Build history of the part. All positions in model axes, mm. Face numbers are marked on the shaded views. Round coordinates to 2 decimals unless told otherwise and drop trailing zeros. Loops run counter-clockwise (first coordinate to the right, second up) from the corner with the lowest first, then second, coordinate; pieces in that order, holes last. Notation, with made-up numbers: (67, 29) -> (116, 29) arc R23 ccw to (116, 40) -> close; hole circle Ø3 at (34, 20). An arc over 180 degrees is marked (long way). Put each result on its own line as item: value. Start each with the question number.
```python
from build123d import *

# Parameters (mm, degrees)
SKETCH_1_W          = 52
SKETCH_1_H          = 28
EXTRUDE_1_DEPTH     = 6
SKETCH_2_W          = 50
SKETCH_2_H          = 26
CUT_EXTRUDE_1_DEPTH = 5
SKETCH_3_W          = 1
SKETCH_3_H          = 26
CUT_EXTRUDE_2_DEPTH = 4
CUT_EXTRUDE_3_REACH = 56.185
SKETCH_6_R          = 1.5
CUT_EXTRUDE_4_DEPTH = 4
EXTRUDE_START       = 3
SKETCH_7_R          = 2.5
SKETCH_7_R_2        = 1.5
SKETCH_7_R_3        = 1
EXTRUDE_3_DEPTH     = 3
CHAMFER_2_SIZE      = 2
CHAMFER_3_SIZE      = 3.5
CHAMFER_3_SIZE2     = 2
FILLET_1_R          = 0.5
FILLET_2_R          = 0.5
EXTRUDE_4_REACH     = 32.799
EXTRUDE_START_2     = -1
SKETCH_9_W          = 0.8
SKETCH_9_H          = 2
CUT_EXTRUDE_5_DEPTH = 1
CHAMFER_4_SIZE      = 1
CHAMFER_4_SIZE_2    = 0.1


# Some blends are built 0.0001 mm under size
with BuildPart() as part:
    # Эскиз1 → Бобышка-Вытянуть1 (new body)
    with BuildSketch(Plane(origin=(0, 0, 0), x_dir=(1, 0, 0), z_dir=(0, 1, 0))):
        Rectangle(SKETCH_1_W, SKETCH_1_H)
    extrude(amount=EXTRUDE_1_DEPTH)

    # Эскиз2 → Вырез-Вытянуть1 (cut)
    with BuildSketch(Plane(origin=(0, 6, 0), x_dir=(1, 0, 0), z_dir=(0, 1, 0))):
        Rectangle(SKETCH_2_W, SKETCH_2_H)
    extrude(amount=-CUT_EXTRUDE_1_DEPTH, mode=Mode.SUBTRACT)

    # Эскиз3 → Вырез-Вытянуть2 (cut)
    with BuildSketch(Plane(origin=(0, 6, 0), x_dir=(1, 0, 0), z_dir=(0, 1, 0))):
        with Locations((25.5, 0)):
            Rectangle(SKETCH_3_W, SKETCH_3_H)
    extrude(amount=-CUT_EXTRUDE_2_DEPTH, mode=Mode.SUBTRACT)

    # Эскиз4 → Вырез-Вытянуть3 (cut, up to next)
    with BuildSketch(Plane.ZY.offset(26), mode=Mode.PRIVATE) as cut_extrude_3_sk1:
        with BuildLine():
            Line((-2.5, 8), (2.5, 8))
            ThreePointArc((2.5, 8), (4, 6.5), (2.5, 5))
            Line((2.5, 5), (-2.5, 5))
            ThreePointArc((-2.5, 5), (-4, 6.5), (-2.5, 8))
        make_face()
    cut_extrude_3_tool1 = extrude(cut_extrude_3_sk1.sketch, amount=-CUT_EXTRUDE_3_REACH, mode=Mode.PRIVATE) & part.part
    add(cut_extrude_3_tool1.solids().sort_by_distance((-26, 6.5, 0))[0], mode=Mode.SUBTRACT)

    # Эскиз6 → Вырез-Вытянуть4 (cut)
    with BuildSketch(Plane(origin=(0, 1, 0), x_dir=(1, 0, 0), z_dir=(0, 1, 0))):
        with Locations(Location((-18.5, 9.5, 0), (0, 0, 270))):
            Circle(SKETCH_6_R)
    extrude(amount=-CUT_EXTRUDE_4_DEPTH, mode=Mode.SUBTRACT)

    # Эскиз7 → Бобышка-Вытянуть3 (add)
    # profile 1 of 2: a face of its own
    with BuildSketch(Plane(origin=(0, 1, 0), x_dir=(1, 0, 0), z_dir=(0, 1, 0)).offset(EXTRUDE_START)):
        with Locations(Location((-18.5, 9.5, 0), (0, 0, 270))):
            Circle(SKETCH_7_R)
        with Locations(Location((-18.5, 9.5, 0), (0, 0, 270))):
            Circle(SKETCH_7_R_2, mode=Mode.SUBTRACT)
    # profile 2 of 2: a face of its own
    with BuildSketch(Plane(origin=(0, 1, 0), x_dir=(1, 0, 0), z_dir=(0, 1, 0)).offset(EXTRUDE_START)):
        with Locations(Location((-23, -11, 0), (0, 0, 270))):
            Circle(SKETCH_7_R_3)
    extrude(amount=-EXTRUDE_3_DEPTH)

    # Фаска2
    # the kernel refuses this chamfer: 2 mm, written as the material it adds along each edge
    with BuildSketch(Plane(origin=(-18.5, 1, -9.5), x_dir=(0, 0, 1), z_dir=(-1, 0, 0))) as chamfer_2_piece_1:
        Polygon((2.5 + CHAMFER_2_SIZE, 0), (2.5, CHAMFER_2_SIZE), (2.5, 0), align=None)
    revolve(axis=Axis((-18.5, 1, -9.5), (0, 1, 0)))

    # Фаска3
    chamfer_3_edges = [part.edges().sort_by_distance(p)[0] for p in [
        (-18.5, 0, -11),
    ]]
    chamfer_3_side = [part.faces().sort_by_distance(p)[0] for p in [
        (-18.5, 2, -11),
    ]]
    chamfer(chamfer_3_edges, length=CHAMFER_3_SIZE, length2=CHAMFER_3_SIZE2, reference=chamfer_3_side[0])

    # Скругление1
    fillet_1_edges = [part.edges().sort_by_distance(p)[0] for p in [
        (-25, 1, 0),
        (4.664213562, 1, -13),
        (-23.164213562, 1, -13),
        (25, 1, 0),
        (0, 1, 13),
        (-22.742640687, 1, -8),
        (0, 0, -14),
        (-26, 0, 0),
        (0, 0, 14),
        (26, 0, 0),
        (-18.5, 0, -13),
        (-18.5, 4, -12),
        (-18.5, 3, -12),
        (25, 1.5, -13),
        (25, 1.5, 13),
        (26, 3, -14),
        (-26, 3, -14),
        (-26, 3, 14),
        (-18.5, 3.5, -11),
    ]]
    fillet(fillet_1_edges, radius=FILLET_1_R)

    # Скругление2
    fillet_2_edges = [part.edges().sort_by_distance(p)[0] for p in [
        (-23, 1, 10),
    ]]
    fillet(fillet_2_edges, radius=FILLET_2_R - 0.0001)  # a hair under: the kernel refuses the full size

    # Эскиз9 → Бобышка-Вытянуть4 (add, up to next)
    with BuildSketch(Plane(origin=(0, 4, 0), x_dir=(1, 0, 0), z_dir=(0, 1, 0)).offset(EXTRUDE_START_2), mode=Mode.PRIVATE) as extrude_4_sk1:
        with Locations((-23, -12)):
            Rectangle(SKETCH_9_W, SKETCH_9_H)
    extrude_4_tool1 = extrude(extrude_4_sk1.sketch, amount=-EXTRUDE_4_REACH, mode=Mode.PRIVATE) - part.part
    # Эскиз9 → Бобышка-Вытянуть4 (add, up to next)
    with BuildSketch(Plane(origin=(0, 4, 0), x_dir=(1, 0, 0), z_dir=(0, 1, 0)).offset(EXTRUDE_START_2), mode=Mode.PRIVATE) as extrude_4_sk2:
        Polygon((-25, -11), (-25, -11.4), (-23, -11.4), (-23, -11), (-23, -10.6), (-25, -10.6), align=None)
    extrude_4_tool2 = extrude(extrude_4_sk2.sketch, amount=-EXTRUDE_4_REACH, mode=Mode.PRIVATE) - part.part
    add(extrude_4_tool1.solids().sort_by_distance((-23, 3, 12))[0])
    add(extrude_4_tool2.solids().sort_by_distance((-24, 3, 11))[0])

    # Эскиз10 → Вырез-Вытянуть5 (cut)
    with BuildSketch(Plane(origin=(0, 6, 0), x_dir=(1, 0, 0), z_dir=(0, 1, 0))):
        Polygon((26, 13), (26, 13.5), (-25.5, 13.5), (-25.5, -13.5), (26, -13.5), (26, -13), (-25, -13), (-25, 13), align=None)
    extrude(amount=-CUT_EXTRUDE_5_DEPTH, mode=Mode.SUBTRACT)

    # Фаска4
    # the kernel refuses this chamfer: 1, 0.1 mm, written as the material it takes off along each edge
    with BuildSketch(Plane(origin=(-25.5, 6, -16.099522763), x_dir=(0, -1, 0), z_dir=(0, 0, 1))) as chamfer_4_piece_1_section:
        Polygon((CHAMFER_4_SIZE, 0), (0, -CHAMFER_4_SIZE_2), (0, 0), align=None)
    chamfer_4_piece_1 = extrude(amount=14.784831964, mode=Mode.PRIVATE)
    chamfer_4_piece_1 = split(chamfer_4_piece_1, bisect_by=Plane(origin=(-25.5, 6.247477501, -13.62474775), z_dir=(0, 0.09950371902099857, 0.9950371902099893)), keep=Keep.TOP, mode=Mode.PRIVATE)
    add(chamfer_4_piece_1, mode=Mode.SUBTRACT)
    with BuildSketch(Plane(origin=(28.599522763, 6, -13.5), x_dir=(0, -1, 0), z_dir=(-1, 0, 0))) as chamfer_4_piece_2_section:
        Polygon((CHAMFER_4_SIZE, 0), (0, -CHAMFER_4_SIZE_2), (0, 0), align=None)
    chamfer_4_piece_2 = extrude(amount=56.699045526, mode=Mode.PRIVATE)
    chamfer_4_piece_2 = split(chamfer_4_piece_2, bisect_by=Plane(origin=(-25.063371062, 0.633710618, -13.5), z_dir=(0.995037190209989, 0.09950371902100032, 0)), keep=Keep.TOP, mode=Mode.PRIVATE)
    add(chamfer_4_piece_2, mode=Mode.SUBTRACT)
    with BuildSketch(Plane(origin=(-28.099522763, 6, 13.5), x_dir=(0, -1, 0), z_dir=(1, 0, 0))) as chamfer_4_piece_3_section:
        Polygon((CHAMFER_4_SIZE, 0), (0, -CHAMFER_4_SIZE_2), (0, 0), align=None)
    chamfer_4_piece_3 = extrude(amount=56.699045526, mode=Mode.PRIVATE)
    chamfer_4_piece_3 = split(chamfer_4_piece_3, bisect_by=Plane(origin=(-25.62474775, 6.247477501, 13.5), z_dir=(0.995037190209989, 0.09950371902100032, 0)), keep=Keep.TOP, mode=Mode.PRIVATE)
    add(chamfer_4_piece_3, mode=Mode.SUBTRACT)
    with BuildSketch(Plane(origin=(-25.5, 6, 1.314690799), x_dir=(0, -1, 0), z_dir=(0, 0, 1))) as chamfer_4_piece_4_section:
        Polygon((CHAMFER_4_SIZE, 0), (0, -CHAMFER_4_SIZE_2), (0, 0), align=None)
    chamfer_4_piece_4 = extrude(amount=14.784831964, mode=Mode.PRIVATE)
    chamfer_4_piece_4 = split(chamfer_4_piece_4, bisect_by=Plane(origin=(-25.5, 4.783632752, 13.478363275), z_dir=(0, 0.09950371902099857, -0.9950371902099893)), keep=Keep.TOP, mode=Mode.PRIVATE)
    add(chamfer_4_piece_4, mode=Mode.SUBTRACT)


solid = part.part
```
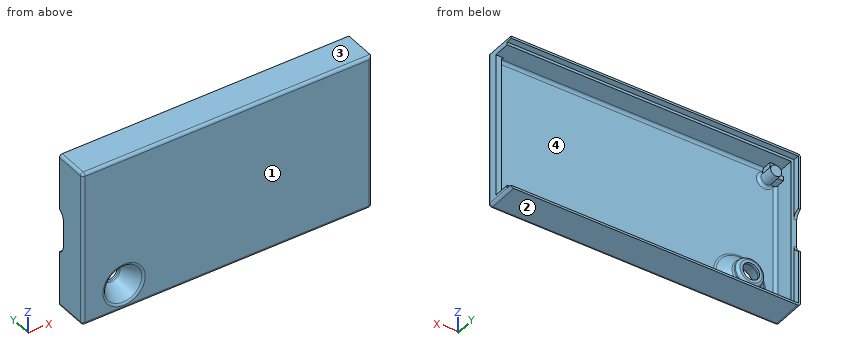
Item 1: Wall check: line 1 (Z direction, x = -10, y = 2.5); line 2 (X direction, y = 3.9, z = -9.5); line 3 (X direction, y = 1.75, z = 9.25). Give the ranges that are in metal, low to high. Write a range as from..to.
Item 2: Cut at B-B on x = -11.5. Write the cut outline in (y, z), then the cut area to 3 significant figures.
Item 3: Cut at D-D on z = 9. Write the cut outline in (x, y).
Item 4: Drop flat-ended pins along their axis: pin 1 (4.5 mm diameter, centred on x = -18, z = -8.5, fed in from +Y); pin 2 (4 mm diameter, centred on x = 12.5, z = 3, fed in from +Y); pin 3 (0.9 mm diameter, centred on x = -23, z = 12.5, fed in from +Y). Give the stop position or say it passes through.
Item 5: Pull direction Z, two halves, no side cores. Call the marked faces 1, 2, 3 and 4: +Z half, -Z half, draft (parallel to the pull), parting line (faces both ways), or undercut.
Item 6: Cut at C-C on z = -0.5. Write the cut outline in (x, y).
Item 7: Cut at A-A on y = 5.5. Write the cut outline in (x, z).
Ans:
1. line 1: z = -14..-13, 13..14
1. line 2: x = -26..-25, -20.8..-20, -17..-16.2
1. line 3: x = -26..-25, 25..26
2. outline: (0, -13.5) arc R0.5 ccw to (0.5, -14) -> (6, -14) -> (6, -13.6) -> (5, -13.5) -> (5, -13) -> (1.5, -13) arc R0.5 cw to (1, -12.5) -> (1, 12.5) arc R0.5 cw to (1.5, 13) -> (5, 13) -> (5, 13.5) -> (6, 13.6) -> (6, 14) -> (0.5, 14) arc R0.5 ccw to (0, 13.5) -> close
2. area: 36.9 mm2
3. outline: (-26, 0.5) arc R0.5 ccw to (-25.5, 0) -> (25.5, 0) arc R0.5 ccw to (26, 0.5) -> (26, 2) -> (25, 2) -> (25, 1.5) arc R0.5 cw to (24.5, 1) -> (-24.5, 1) arc R0.5 cw to (-25, 1.5) -> (-25, 5) -> (-25.5, 5) -> (-25.6, 6) -> (-26, 6) -> close
4. pin 1: stops at y = 4
4. pin 2: stops at y = 1
4. pin 3: stops at y = 3
5. face 1: draft
5. face 2: -Z half
5. face 3: +Z half
5. face 4: undercut
6. outline: (-26, 0.5) arc R0.5 ccw to (-25.5, 0) -> (25.5, 0) arc R0.5 ccw to (26, 0.5) -> (26, 2) -> (25, 2) -> (25, 1.5) arc R0.5 cw to (24.5, 1) -> (-24.5, 1) arc R0.5 cw to (-25, 1.5) -> (-25, 5) -> (-26, 5) -> close
7. outline: (-26, -13.5) arc R0.5 ccw to (-25.5, -14) -> (25.5, -14) arc R0.5 ccw to (26, -13.55) -> (-25.55, -13.55) -> (-25.55, -3.62) -> (-26, -3.62) -> close; (-26, 3.62) -> (-25.55, 3.62) -> (-25.55, 13.55) -> (26, 13.55) -> (26, 14) -> (-25.5, 14) arc R0.5 ccw to (-26, 13.5) -> close
